from build123d import *

# Parameters (mm, degrees)
SKETCH1_W           = 45
SKETCH1_H           = 40
BOSS_EXTRUDE1_DEPTH = 6
SKETCH2_W           = 5
SKETCH2_H           = 5
SKETCH2_H_2         = 7
CUT_EXTRUDE1_DEPTH  = 6
SKETCH3_W           = 5
SKETCH3_H           = 7
SKETCH3_H_2         = 3
CUT_EXTRUDE2_DEPTH  = 6


with BuildPart() as part:
    # Sketch1 → Boss-Extrude1 (new body)
    with BuildSketch(Plane(origin=(0, 0, 0), x_dir=(0, 0, -1), z_dir=(1, 0, 0))):
        with Locations((0.079787234, -3.244680851)):
            Rectangle(SKETCH1_W, SKETCH1_H)
    extrude(amount=BOSS_EXTRUDE1_DEPTH)

    # Sketch2 → Cut-Extrude1 (cut)
    with BuildSketch(Plane(origin=(6, 0, 0), x_dir=(0, 0, -1), z_dir=(1, 0, 0))):
        with Locations((-19.920212766, 9.255319149)):
            Rectangle(SKETCH2_W, SKETCH2_H)
        with Locations((-19.920212766, -1.744680851)):
            Rectangle(SKETCH2_W, SKETCH2_H_2)
        with Locations((-19.920212766, -10.744680851)):
            Rectangle(SKETCH2_W, SKETCH2_H)
    extrude(amount=-CUT_EXTRUDE1_DEPTH, mode=Mode.SUBTRACT)

    # Sketch3 → Cut-Extrude2 (cut)
    with BuildSketch(Plane(origin=(6, 0, 0), x_dir=(0, 0, -1), z_dir=(1, 0, 0))):
        with Locations((20.079787234, 13.255319149)):
            Rectangle(SKETCH3_W, SKETCH3_H)
        with Locations((20.079787234, -3.244680851)):
            Rectangle(SKETCH3_W, SKETCH3_H_2)
        with Locations((20.079787234, -19.744680851)):
            Rectangle(SKETCH3_W, SKETCH3_H)
    extrude(amount=-CUT_EXTRUDE2_DEPTH, mode=Mode.SUBTRACT)


solid = part.part
Can you work these out from the model? Positions are in its coordinate system, mm. A direction names the side the tool comes from. Coordinates: 2 decimals unless noted, no trailing zeros. Write each loop counter-clockwise with the first axis right and the second up, starting at its lowest first coordinate (ties: lowest second). Pieces come first, ordered by that corner, then holes. Notation, with made-up numbers: (30.25, -39) - (68.25, -39) arc R22 cw to (68.25, -8) - close; hole circle Ø11 at (-13.5, 69.5). An arc over 180 degrees is marked (long way). Return JSON: item names as keys, results as strings. Group by question number.
Item 1: If we section it at A-A (z = -19): Write out the boundary of the cut face in (x, y).
Item 2: Which directions (+Z, -Z, +X, -X, +Y, -Y) give clear straight access to the entire face, cutting with the end or side of a thin tool? Please do faces 1 (the face through (3, 9.755, -20)), 2 (the face through (3, 11.755, 20)), 3 (the face through (3, -3, -17.58)).
Item 3: If we section it at C-C (y = 14): Write out the boundary of the cut face in (x, z), then the cut area to 3 significant figures.
Item 4: We'd pull the mould along Y, two halves only. Please class faces 4 (the face through (3, -16.245, -20)), 5 (the face through (6, -3, 0)), 6 (the face through (3, 6.755, 20)): pulls with the +Y half, pulls with the -Y half, needs draft (parallel to the pull), parting line crosses it, or undercut.
Item 5: Please list where these lines run through material, in increasing order: probe 1 along Y at (x, z) = (4.6, 19); probe 2 along Y at (x, z) = (1.6, -18); probe 3 along Z at (x, y) = (3.65, 1).
Item 6: I'm going to push a flat-ended pin straight in: pin 1 Ø3 at (x, y) = (2.5, -20) entering from -Z. Where does the tip first touch, or does it pass through?
Item 7: If we section it at B-B (x = 4.35): Write out the boundary of the cut face in (y, z), then the cut area to 3 significant figures.
Return value:
{
 "1": {"outline": "(0, -16.24) - (6, -16.24) - (6, -4.74) - (0, -4.74) - close; (0, -1.74) - (6, -1.74) - (6, 9.76) - (0, 9.76) - close"},
 "2": {"face 1": "-Z, +X, -X, +Y", "face 2": "+Z, +X, -X", "face 3": "-Z, +X, -X"},
 "3": {"outline": "(0, -17.58) - (6, -17.58) - (6, 22.42) - (0, 22.42) - close", "area": "240 mm^2"},
 "4": {"face 4": "pulls with the -Y half", "face 5": "needs draft", "face 6": "undercut"},
 "5": {"probe 1": "y = -23.24 to -13.24, -8.24 to -5.24, 1.76 to 6.76, 11.76 to 16.76", "probe 2": "y = -16.24 to -4.74, -1.74 to 9.76", "probe 3": "z = -22.58 to 17.42"},
 "6": {"pin 1": "stops at z = -17.58"},
 "7": {"outline": "(-23.24, -17.58) - (-16.24, -17.58) - (-16.24, -22.58) - (-4.74, -22.58) - (-4.74, -17.58) - (-1.74, -17.58) - (-1.74, -22.58) - (9.76, -22.58) - (9.76, -17.58) - (16.76, -17.58) - (16.76, 22.42) - (11.76, 22.42) - (11.76, 17.42) - (6.76, 17.42) - (6.76, 22.42) - (1.76, 22.42) - (1.76, 17.42) - (-5.24, 17.42) - (-5.24, 22.42) - (-8.24, 22.42) - (-8.24, 17.42) - (-13.24, 17.42) - (-13.24, 22.42) - (-23.24, 22.42) - close", "area": "1,630 mm^2"}
}
